```python
from build123d import *

# Parameters (mm, degrees)
SKETCH1_R           = 2.4892
BOSS_EXTRUDE1_DEPTH = 3.175
SKETCH2_R           = 2.4892
CUT_EXTRUDE1_DEPTH  = 4.175


with BuildPart() as part:
    # Sketch1 → Boss-Extrude1 (new body)
    with BuildSketch(Plane(origin=(0, 0, 0), x_dir=(1, 0, 0), z_dir=(0, 1, 0))):
        with BuildLine():
            Line((-101.6, 10.2108), (-101.6, 0))
            Line((-101.6, 0), (101.6, 0))
            Line((101.6, 0), (101.6, 10.2108))
            ThreePointArc((101.6, 10.2108), (99.1108, 12.7), (101.6, 15.1892))
            Line((101.6, 15.1892), (101.6, 88.9))
            Line((101.6, 88.9), (76.2, 88.9))
            Line((76.2, 88.9), (76.2, 25.4))
            Line((76.2, 25.4), (-76.2, 25.4))
            Line((-76.2, 25.4), (-76.2, 88.9))
            Line((-76.2, 88.9), (-101.6, 88.9))
            Line((-101.6, 88.9), (-101.6, 15.1892))
            ThreePointArc((-101.6, 15.1892), (-99.8398698, 14.4601302), (-99.1108, 12.7))
            ThreePointArc((-99.1108, 12.7), (-99.8398698, 10.9398698), (-101.6, 10.2108))
        make_face()
        with Locations((-76.2, 12.7)):
            Circle(SKETCH1_R, mode=Mode.SUBTRACT)
        with Locations((-50.8, 12.7)):
            Circle(SKETCH1_R, mode=Mode.SUBTRACT)
        with Locations((-25.4, 12.7)):
            Circle(SKETCH1_R, mode=Mode.SUBTRACT)
        with Locations((0, 12.7)):
            Circle(SKETCH1_R, mode=Mode.SUBTRACT)
        with Locations((25.4, 12.7)):
            Circle(SKETCH1_R, mode=Mode.SUBTRACT)
        with Locations((50.8, 12.7)):
            Circle(SKETCH1_R, mode=Mode.SUBTRACT)
        with Locations((76.2, 12.7)):
            Circle(SKETCH1_R, mode=Mode.SUBTRACT)
    extrude(amount=BOSS_EXTRUDE1_DEPTH)

    # Sketch2 → Cut-Extrude1 (cut, through all)
    with BuildSketch(Plane(origin=(0, 3.175, 0), x_dir=(1, 0, 0), z_dir=(0, 1, 0))):
        with Locations((-88.9, 50.8)):
            Circle(SKETCH2_R)
        with Locations((-88.9, 76.2)):
            Circle(SKETCH2_R)
        with Locations((88.9, 76.2)):
            Circle(SKETCH2_R)
        with Locations((88.9, 50.8)):
            Circle(SKETCH2_R)
    extrude(amount=-CUT_EXTRUDE1_DEPTH, mode=Mode.SUBTRACT)


solid = part.part
```
The model under review builds one solid part; all positions refer to its coordinate system, in mm. Round coordinates to 2 decimals unless told otherwise and drop trailing zeros. Order: outer loops, then holes, each group sorted by start corner. A loop starts at its lowest first (then second) coordinate and runs counter-clockwise, first axis right, second up. Notation, with made-up numbers: (-15.5, 77.25) -> (-8.5, 77.25) arc R12 cw to (-8.5, 92.25) -> close; hole circle Ø2 at (87.25, 60.25). An arc over 180 degrees is marked (long way). Use a Markdown table: item, result.
Q1. For line 1 (Z direction, x = 88.9, y = 2.2); line 2 (X direction, y = 2.55, z = -50.8); line 3 (X direction, y = 2.1, z = -52), list the stretches that pass through material, from the lowest coordinate up.
Values:
| item | result |
|---|---|
| line 1 | z = -88.9 to -78.69, -73.71 to -53.29, -48.31 to 0 |
| line 2 | x = -101.6 to -91.39, -86.41 to -76.2, 76.2 to 86.41, 91.39 to 101.6 |
| line 3 | x = -101.6 to -91.08, -86.72 to -76.2, 76.2 to 86.72, 91.08 to 101.6 |
Q2. We need section C-C on x = 0. Write out the cut boundary in (y, z) (3 decimals).
Values:
| item | result |
|---|---|
| outline | (0, -25.4) -> (3.175, -25.4) -> (3.175, -15.189) -> (0, -15.189) -> close; (0, -10.211) -> (3.175, -10.211) -> (3.175, 0) -> (0, 0) -> close |
Q3. We need section B-B on z = -58.5. Write out the cut boundary in (x, y) (3 decimals).
Values:
| item | result |
|---|---|
| outline | (-101.6, 0) -> (-76.2, 0) -> (-76.2, 3.175) -> (-101.6, 3.175) -> close; (76.2, 0) -> (101.6, 0) -> (101.6, 3.175) -> (76.2, 3.175) -> close |
Q4. We need section A-A on z = -76.2. Write out the cut boundary in (x, y) (3 decimals).
Values:
| item | result |
|---|---|
| outline | (-101.6, 0) -> (-91.389, 0) -> (-91.389, 3.175) -> (-101.6, 3.175) -> close; (-86.411, 0) -> (-76.2, 0) -> (-76.2, 3.175) -> (-86.411, 3.175) -> close; (76.2, 0) -> (86.411, 0) -> (86.411, 3.175) -> (76.2, 3.175) -> close; (91.389, 0) -> (101.6, 0) -> (101.6, 3.175) -> (91.389, 3.175) -> close |
Q5. Mouldability with a two-part tool opening along Z and no side actions: class faces 1 (the cylindrical face through (-23.026, 1.565, -13.448)), 2 (the cylindrical face through (-78.687, 1.565, -12.809)), 3 (the flat face through (-1, 3.175, -25)) as +Z half, -Z half, draft (parallel to the pull), parting line (faces both ways), or undercut.
Values:
| item | result |
|---|---|
| face 1 | undercut |
| face 2 | undercut |
| face 3 | draft |
Q6. We need section D-D on y = 2.3. State how many separate pieces and enclosed holes the cut face has, then the cut area to 3 significant figures.
Values:
| item | result |
|---|---|
| separate pieces | 1 |
| enclosed holes | 11 |
| area | 8,150 mm^2 |
Q7. Clearance check with a flat-ended pin moving along its axis: P1, Ø1, axis at x = 16, y = 1, coming from the -Z side. State where the tip first meets the part, or that it passes through.
Values:
| item | result |
|---|---|
| P1 | stops at z = -25.4 |
